Source: CAD feature listing. Evaluate the final solid. Frame: model axes, mm. A direction names the side the tool comes from. Give positions to 0.01 mm unless a question says otherwise; leave off trailing zeros. Write each loop counter-clockwise with the first axis right and the second up, starting at its lowest first coordinate (ties: lowest second). Pieces come first, ordered by that corner, then holes.
Autodesk Inventor part; units mm, degrees
ref_plane "YZ Plane" through (0, 0, 0) normal (1, 0, 0) x (0, 1, 0)
ref_plane "XZ Plane" through (0, 0, 0) normal (0, 1, 0) x (-1, 0, 0)
ref_plane "XY Plane" through (0, 0, 0) normal (0, 0, 1) x (1, 0, 0)
sketch "Sketch1" plane through (0, 0, 0) normal (0, 0, 1) x (1, 0, 0)
  line L0 (0, 0) -> (-50.8, 0)
  line L1 (-50.8, 0) -> (-50.8, -12.7)
  line L2 (-50.8, -12.7) -> (-38.1, -12.7)
  line L3 (-12.0663, -25.4) -> (-12.0663, -35.56)
  line L4 (-5, -35.56) -> (-5, -4.064)
  line L5 (-5, -4.064) -> (0, -4.064)
  line L6 (0, -4.064) -> (0, 0)
  line L7 (-12.0663, -35.56) -> (-5, -35.56)
  line L8 (-38.1, -12.7) -> (-12.0663, -12.7)
  line L9 (-12.0663, -12.7) -> (-12.0663, -25.4)
  dimension "d0" = 50.8
  dimension "d1" = 5
  dimension "d2" = 12.0663
  dimension "d13" = 22.86
  dimension "d15" = 31.496
revolve "Revolution1" add sketch "Sketch1" angle 360 about axis through (0, -4.064, 0) along (0, 1, 0)
sketch "Sketch5" plane through (0, 0, 0) normal (0, 1, 0) x (1, 0, 0)
  circle A0 centre (0, 0) radius 5
  line L0 (9.815, 0) -> (4.9075, -8.5)
  line L1 (4.9075, -8.5) -> (-4.9075, -8.5)
  line L2 (-4.9075, -8.5) -> (-9.815, 0)
  line L3 (-9.815, 0) -> (-4.9075, 8.5)
  line L4 (-4.9075, 8.5) -> (4.9075, 8.5)
  line L5 (4.9075, 8.5) -> (9.815, 0)
  point P0 (0, 0)
  point P1 (0, 0)
  dimension "d16" = 17
extrude "Extrusion1" cut sketch "Sketch5" against normal blind 12.7 contours A0 | L0 L1 L2 L3 L4 L5
sketch "Sketch7" plane through (0, -12.7, 0) normal (0, -1, 0) x (1, 0, 0)
  circle A0 centre (0, 0) radius 50.8
  line L0 (47.0929, -19.05) -> (85.1929, -19.05)
  line L1 (85.1929, -19.05) -> (85.1929, -31.75)
  line L2 (85.1929, -31.75) -> (39.6557, -31.75)
  circle A1 centre (0, 0) radius 5 construction
  line L3 (0, 0) -> (5, 0) construction
  line L4 (50.8, 0) -> (83.823, 0) construction
  dimension "d23" = 38.1
  dimension "d24" = 12.7
  dimension "d25" = 19.05
extrude "Extrusion3" add sketch "Sketch7" against normal blind 12.7 contours A0 L0 L1 L2
sketch "Sketch8" plane through (39.6557, 0, -31.75) normal (0, 1, 0) x (1, 0, 0)
  line L0 (45.5371, -12.7) -> (45.5371, 0)
  line L1 (45.5371, 0) -> (0, 0)
  line L2 (7.4371, -12.7) -> (45.5371, -12.7)
  line L3 (35.8511, -107.95) -> (35.8511, 44.45)
  line L4 (26.3261, -107.95) -> (26.3261, 44.45)
  line L5 (45.5371, -12.7) -> (23.3121, -12.7)
  line L6 (23.3121, -12.7) -> (23.3121, 0)
  line L7 (23.3121, 0) -> (45.5371, 0)
  line L8 (45.5371, 0) -> (45.5371, -12.7)
  point P0 (-39.6557, -31.75)
  point P1 (23.3121, 0)
  point P2 (23.3121, -12.7)
  dimension "d28" = 22.225
extrude "Extrusion4" add sketch "Sketch8" along normal blind 19.05
sketch "Sketch9" plane through (85.1929, -12.7, -31.75) normal (0, 0, -1) x (-1, 0, 0)
  line L0 (22.225, 12.7) -> (22.225, 31.75)
  line L1 (0, 31.75) -> (22.225, 31.75)
  arc A0 (38.6742, 14.3599) -> (35.4992, 14.3599) centre (37.0867, 18.85) ccw
  line L2 (0, 0) -> (0, 31.75)
  circle A1 centre (37.0867, 18.85) radius 4.953
  point P0 (85.1929, 12.7)
  dimension "d31" = 9.906
extrude "Extrusion5" cut sketch "Sketch9" against normal through all
mirror "Mirror1" about plane through (0, 0, 0) normal (0, 0, 1) of "Extrusion4", "Extrusion5", "Extrusion3"
sketch "Sketch10" plane through (39.6557, -12.7, -31.75) normal (0, -1, 0) x (1, 0, 0)
  arc A0 (7.4371, 12.7) -> (7.4371, 50.8) centre (-39.6557, 31.75) ccw
  line L0 (45.5371, 50.8) -> (7.4371, 50.8)
  line L1 (45.5371, 12.7) -> (7.4371, 12.7)
  arc A1 (7.4371, 12.7) -> (7.4371, 50.8) centre (-39.6557, 31.75) ccw
  line L2 (7.4371, 50.8) -> (45.5371, 50.8)
  line L3 (45.5371, 0) -> (45.5371, 12.7)
  line L4 (45.5371, 50.8) -> (45.5371, 12.7)
  line L5 (45.5371, 12.7) -> (7.4371, 12.7)
extrude "Extrusion6" add sketch "Sketch10" against normal blind 6.35
sketch "Sketch11" plane through (85.1929, -12.7, -31.75) normal (1, 0, 0) x (0, 0, -1)
  line L0 (-63.5, 0) -> (-63.5, 31.75)
  line L1 (-50.8, 31.75) -> (-63.5, 31.75)
  line L2 (-12.7, 31.75) -> (0, 31.75)
  line L3 (0, 0) -> (0, 31.75)
  line L4 (0, 0) -> (-63.5, 0)
  line L5 (-63.5, 31.75) -> (0, 31.75)
  line L6 (0, 31.75) -> (0, 0)
  line L7 (0, 0) -> (-63.5, 0)
  line L8 (-63.5, 0) -> (-63.5, 31.75)
  point P0 (-31.75, 12.7)
  point P1 (-12.7, 31.75)
  point P2 (-50.8, 31.75)
extrude "Extrusion7" add sketch "Sketch11" along normal blind 6.35
sketch "Sketch12" plane through (39.6557, 19.05, -31.75) normal (0, 1, 0) x (1, 0, 0)
  point P0 (-39.6557, -31.75)
equation "\"d0\" = topPartRadius"
equation "\"d2\" = stemRadius"
equation "\"d13\" = stemHeight"
equation "\"d15\" = internalHoleDepth"
equation "\"topPartRadius\" = 0.5 * topPartDiameter"
equation "\"totalHeight\" = 35.56"
equation "\"stemRadius\" = 12.06627"
equation "\"stemHeight\" = 22.86"
equation "\"internalHoleDepth\" = 31.496"
equation "\"topPartDiameter\" = 101.6"
properties part number "celestronTripodAdapter" material "PC/ABS Plastic"
1. Cut plane C-C, the plane x = 77. Return the cut outline in (y, z), then the cut area to 3 significant figures.
2. Line query: L1, parallel to Z at x = 0, y = -19; L2, parallel to Y at x = -5.5, z = 19; L3, parallel to X at y = 15, z = 11. Output: solid intervals per line, ascending.
3. Access query for faces 1 (the flat face through (91.543, 3, 0)), 2 (the flat face through (4, -12.7, -4)), 3 (the flat face through (71, -1, -31.75)), 4 (the flat face through (7, 0, 12)). Directions: +Z, -Z, +X, -X, +Y, -Y. A direction counts if a zero-diameter tool reaches every point of the face in a straight line with its end or side. Return the directions, or none.
4. Cut plane B-B, the plane y = 1.5. Return the cut outline in (x, z), then the cut area to 3 significant figures.
5. Contact query for flat-ended pins moving along their axis: P1, Ø5, axis at x = -4, z = 3.5, coming from the +Y side; P2, Ø12.5, axis at x = 66, y = 10, coming from the -Z side; P3, Ø6, axis at x = 4.5, z = 16.5, coming from the -Y side. Output: stop coordinate, or through.
6. Mould query, pull axis X, two halves, no side actions, for faces 5 (the flat face through (71, -1, 31.75)), 6 (the flat face through (-7.396, -6.261, -4.19)), 7 (the flat face through (-7.327, -6.261, 4.31)), 8 (the flat face through (62.968, 9, -25)). Classes: +X half, -X half, draft (parallel to the pull), parting line (faces both ways), or undercut.
7. Cut plane D-D, the plane y = -22. Return the cut outline in (x, z), then the cut area to 3 significant figures.
8. Cut plane A-A, the plane x = 0. Return the cut outline in (y, z), then the cut area to 3 significant figures.
Response values:
1. outline: (-12.7, -31.75) - (19.05, -31.75) - (19.05, -19.05) - (-6.35, -19.05) - (-6.35, 19.05) - (19.05, 19.05) - (19.05, 31.75) - (-12.7, 31.75) - close
1. area: 1,050 mm2
2. L1: z = -12.07 to -5, 5 to 12.07
2. L2: y = -12.7 to 0
2. L3: x = 85.19 to 91.54
3. face 1: +Z, -Z, +X, +Y, -Y
3. face 2: +Y
3. face 3: -Z, +X, +Y, -Y
3. face 4: +Z, -Z, -X, +Y
4. outline: (62.97, -31.75) - (91.54, -31.75) - (91.54, 31.75) - (62.97, 31.75) - (62.97, 19.05) - (85.19, 19.05) - (85.19, -19.05) - (62.97, -19.05) - close
4. area: 968 mm2
5. P1: stops at y = -12.7
5. P2: stops at z = -31.75
5. P3: stops at y = -12.7
6. face 5: draft
6. face 6: undercut
6. face 7: undercut
6. face 8: -X half
7. outline: circle Ø24.13 at (0, 0); hole circle Ø10 at (0, 0)
7. area: 379 mm2
8. outline: (-35.56, -12.07) - (-12.7, -12.07) - (-12.7, -50.8) - (0, -50.8) - (0, -8.5) - (-12.7, -8.5) - (-12.7, -5) - (-35.56, -5) - close; (-35.56, 5) - (-12.7, 5) - (-12.7, 8.5) - (0, 8.5) - (0, 50.8) - (-12.7, 50.8) - (-12.7, 12.07) - (-35.56, 12.07) - close
8. area: 1,400 mm2
